Could you check a few things on this model? Use its own coordinates, in mm. Face numbers are marked on the shaded views. Give positions to 0.01 mm unless a question says otherwise; leave off trailing zeros. Loops run counter-clockwise (first coordinate to the right, second up) from the corner with the lowest first, then second, coordinate; pieces in that order, holes last.
1. Imagine slicing it at A-A (z = 0). List the corners of the cut face in (x, y) for me.
2. Imagine slicing it at C-C (x = -47.5). List the corners of the cut face in (y, z) for me, plus the area to 3 significant figures.
3. I need wall thicknesses on line 1 along X through (y, z) = (17.5, 16.7); line 2 along X through (y, z) = (16.6, -61.5); line 3 along Y through (x, z) = (-8, -17.05). Which ranges of each line are inside material? Lowest first, please.
4. Imagine slicing it at B-B (x = -27). List the corners of the cut face in (y, z) for me, plus the area to 3 significant figures.
5. For P1, Ø10, axis at y = 10.5, z = -67.5, coming from the -X side; P2, Ø5, axis at x = -3, y = 16.5, coming from the +Z side; P3, Ø1.4, axis at x = -8, y = 17.5, coming from the +Z side; P4, Ø2, axis at x = 8.5, y = 11.5, coming from the -Z side, each with a flat end and sliding along its axis, tell me the tip position at first contact or that it passes through.
6. Thinking about a two-plate mould opening in Z: for the marked faces 1 and 2, which applies, +Z half, -Z half, draft (parallel to the pull), parting line (faces both ways), or undercut?
7. Imagine slicing it at D-D (x = 58.5). List the corners of the cut face in (y, z) for me.
```python
from build123d import *

# Parameters (mm, degrees)
SKETCH1_R                                           = 37.65
SKETCH1_R_2                                         = 32.65
BOSS_EXTRUDE1_DEPTH                                 = 10
BOSS_EXTRUDE2_START                                 = -4
SKETCH2_R                                           = 32.65
SKETCH2_R_2                                         = 29.65
BOSS_EXTRUDE2_DEPTH                                 = 4
SKETCH3_R                                           = 85
BOSS_EXTRUDE3_DEPTH                                 = 5
SKETCH4_W                                           = 27
SKETCH4_H                                           = 6
BOSS_EXTRUDE4_DEPTH                                 = 6
FILLET1_R                                           = 3
SKETCH6_R                                           = 2.25
CUT_EXTRUDE1_DEPTH                                  = 3
CSK_FOR_M2_COUNTERSUNK_FLAT_HEAD_SCREW1_D           = 2.4
CSK_FOR_M2_COUNTERSUNK_FLAT_HEAD_SCREW1_CSINK_D     = 4.4
CSK_FOR_M2_COUNTERSUNK_FLAT_HEAD_SCREW1_CSINK_ANGLE = 90
FILLET1_OF_MIRROR1_R                                = 3
SKETCH8_R                                           = 2.25
CUT_EXTRUDE2_DEPTH                                  = 5
SKETCH11_W                                          = 6
SKETCH11_H                                          = 16
BOSS_EXTRUDE5_DEPTH                                 = 3
CSK_FOR_M2_COUNTERSUNK_FLAT_HEAD_SCREW2_D           = 2.4
CSK_FOR_M2_COUNTERSUNK_FLAT_HEAD_SCREW2_CSINK_D     = 4.4
CSK_FOR_M2_COUNTERSUNK_FLAT_HEAD_SCREW2_CSINK_ANGLE = 90
LPATTERN1_COUNT                                     = 2
LPATTERN1_PITCH                                     = 16
LPATTERN1_COPY_1_SKETCH_R                           = 2.25
LPATTERN1_COPY_1_DEPTH                              = 5
LPATTERN1_COPY_2_SKETCH_W                           = 6
LPATTERN1_COPY_2_SKETCH_H                           = 16
LPATTERN1_COPY_2_DEPTH                              = 3
LPATTERN1_COPY_3_D                                  = 2.4
LPATTERN1_COPY_3_CSINK_D                            = 4.4
LPATTERN1_COPY_3_CSINK_ANGLE                        = 90
CUT_EXTRUDE3_DEPTH                                  = 122.140414396
CUT_EXTRUDE3_DEPTH_BACK                             = 122.140414396
SKETCH12_R                                          = 12


with BuildPart() as part:
    # Sketch1 → Boss-Extrude1 (new body)
    with BuildSketch(Plane(origin=(0, 0, 0), x_dir=(1, 0, 0), z_dir=(0, 1, 0))):
        with Locations(Location((0, 0, 0), (0, 0, 270))):
            Circle(SKETCH1_R)
        with Locations(Location((0, 0, 0), (0, 0, 270))):
            Circle(SKETCH1_R_2, mode=Mode.SUBTRACT)
    extrude(amount=BOSS_EXTRUDE1_DEPTH)

    # Sketch2 → Boss-Extrude2 (add)
    with BuildSketch(Plane(origin=(0, 10, 0), x_dir=(1, 0, 0), z_dir=(0, 1, 0)).offset(BOSS_EXTRUDE2_START)):
        with Locations(Location((0, 0, 0), (0, 0, 270))):
            Circle(SKETCH2_R)
        with Locations(Location((0, 0, 0), (0, 0, 270))):
            Circle(SKETCH2_R_2, mode=Mode.SUBTRACT)
    extrude(amount=BOSS_EXTRUDE2_DEPTH)

    # Sketch3 → Boss-Extrude3 (add)
    with BuildSketch(Plane(origin=(0, 10, 0), x_dir=(1, 0, 0), z_dir=(0, 1, 0))):
        with Locations(Location((0, 0, 0), (0, 0, 270))):
            Circle(SKETCH3_R)
    extrude(amount=BOSS_EXTRUDE3_DEPTH)

    # Sketch4 → Boss-Extrude4 (add)
    with BuildSketch(Plane(origin=(0, 15, 0), x_dir=(1, 0, 0), z_dir=(0, 1, 0))):
        with Locations((0, 19)):
            Rectangle(SKETCH4_W, SKETCH4_H)
    boss_extrude4 = extrude(amount=BOSS_EXTRUDE4_DEPTH)

    # Fillet1
    fillet1_edges = [part.edges().sort_by_distance(p)[0] for p in [
        (-13.5, 21, -19),
        (13.5, 21, -19),
    ]]
    fillet(fillet1_edges, radius=FILLET1_R)

    # Sketch6 → Cut-Extrude1 (cut)
    with BuildSketch(Plane(origin=(0, 0, -22), x_dir=(-1, 0, 0), z_dir=(0, 0, -1))):
        with Locations((-8, 17.5)):
            Circle(SKETCH6_R)
        with Locations((8, 17.5)):
            Circle(SKETCH6_R)
    cut_extrude1 = extrude(amount=-CUT_EXTRUDE1_DEPTH, mode=Mode.SUBTRACT)

    # CSK for M2 Countersunk Flat Head Screw1 (through all)
    with Locations(Plane(origin=(8, 17.5, -19), x_dir=(-1, 0, 0), z_dir=(0, 0, -1))):
        with Locations((0, 0), (16, 0)):
            csk_for_m2_countersunk_flat_head_screw1 = CounterSinkHole(CSK_FOR_M2_COUNTERSUNK_FLAT_HEAD_SCREW1_D / 2, CSK_FOR_M2_COUNTERSUNK_FLAT_HEAD_SCREW1_CSINK_D / 2, counter_sink_angle=CSK_FOR_M2_COUNTERSUNK_FLAT_HEAD_SCREW1_CSINK_ANGLE)

    # Mirror1: Boss-Extrude4, Cut-Extrude1, CSK for M2 Countersunk Flat Head Screw1 across plane
    add(boss_extrude4.mirror(Plane.XY))
    add(cut_extrude1.mirror(Plane.XY), mode=Mode.SUBTRACT)
    add(csk_for_m2_countersunk_flat_head_screw1.mirror(Plane.XY), mode=Mode.SUBTRACT)

    # Fillet1 of Mirror1
    fillet1_of_mirror1_edges = [part.edges().sort_by_distance(p)[0] for p in [
        (-13.5, 21, 19),
        (13.5, 21, 19),
    ]]
    fillet(fillet1_of_mirror1_edges, radius=FILLET1_OF_MIRROR1_R)

    # Sketch8 → Cut-Extrude2 (cut)
    with BuildSketch(Plane(origin=(0, 10, 0), x_dir=(-1, 0, 0), z_dir=(0, -1, 0))):
        with Locations(Location((13.5, 61.5, 0), (0, 0, 90))):
            Circle(SKETCH8_R)
    cut_extrude2 = extrude(amount=-CUT_EXTRUDE2_DEPTH, mode=Mode.SUBTRACT)

    # Sketch11 → Boss-Extrude5 (add)
    with BuildSketch(Plane(origin=(0, 15, 0), x_dir=(1, 0, 0), z_dir=(0, 1, 0))):
        with Locations((-13.5, 58.5)):
            Rectangle(SKETCH11_W, SKETCH11_H)
    boss_extrude5 = extrude(amount=BOSS_EXTRUDE5_DEPTH)

    # CSK for M2 Countersunk Flat Head Screw2 (through all)
    with Locations(Plane(origin=(-13.5, 15, -61.5), x_dir=(0, 0, -1), z_dir=(0, -1, 0))):
        with Locations((0, 0)):
            csk_for_m2_countersunk_flat_head_screw2 = CounterSinkHole(CSK_FOR_M2_COUNTERSUNK_FLAT_HEAD_SCREW2_D / 2, CSK_FOR_M2_COUNTERSUNK_FLAT_HEAD_SCREW2_CSINK_D / 2, counter_sink_angle=CSK_FOR_M2_COUNTERSUNK_FLAT_HEAD_SCREW2_CSINK_ANGLE)

    # Mirror2: Cut-Extrude2, Boss-Extrude5, CSK for M2 Countersunk Flat Head Screw2 across plane
    add(cut_extrude2.mirror(Plane(origin=(0, 0, 0), x_dir=(0, 0, 1), z_dir=(1, 0, 0))), mode=Mode.SUBTRACT)
    add(boss_extrude5.mirror(Plane(origin=(0, 0, 0), x_dir=(0, 0, 1), z_dir=(1, 0, 0))))
    add(csk_for_m2_countersunk_flat_head_screw2.mirror(Plane(origin=(0, 0, 0), x_dir=(0, 0, 1), z_dir=(1, 0, 0))), mode=Mode.SUBTRACT)

    # LPattern1: Cut-Extrude2, Boss-Extrude5, CSK for M2 Countersunk Flat Head Screw2 ×2
    with Locations(*[(0, 0, i * LPATTERN1_PITCH) for i in range(1, LPATTERN1_COUNT)]):
        add(cut_extrude2, mode=Mode.SUBTRACT)
        add(boss_extrude5)
        add(csk_for_m2_countersunk_flat_head_screw2, mode=Mode.SUBTRACT)

    # LPattern1 copy 1 sketch → LPattern1 copy 1 (cut)
    with BuildSketch(Plane(origin=(0, 10, 16), x_dir=(1, 0, 0), z_dir=(0, -1, 0))):
        with Locations((13.5, -61.5)):
            Circle(LPATTERN1_COPY_1_SKETCH_R)
    extrude(amount=-LPATTERN1_COPY_1_DEPTH, mode=Mode.SUBTRACT)

    # LPattern1 copy 2 sketch → LPattern1 copy 2 (add)
    with BuildSketch(Plane(origin=(0, 15, 16), x_dir=(-1, 0, 0), z_dir=(0, 1, 0))):
        with Locations((-13.5, -58.5)):
            Rectangle(LPATTERN1_COPY_2_SKETCH_W, LPATTERN1_COPY_2_SKETCH_H)
    extrude(amount=LPATTERN1_COPY_2_DEPTH)

    # LPattern1 copy 3 (through all)
    with Locations(Plane(origin=(13.5, 15, -45.5), x_dir=(0, 0, -1), z_dir=(0, -1, 0))):
        with Locations((0, 0)):
            CounterSinkHole(LPATTERN1_COPY_3_D / 2, LPATTERN1_COPY_3_CSINK_D / 2, counter_sink_angle=LPATTERN1_COPY_3_CSINK_ANGLE)

    # Sketch12 → Cut-Extrude3 (cut, two sides: drawn at the far end of the back side and taken through both)
    with BuildSketch(Plane(origin=(0, 15, 0), x_dir=(1, 0, 0), z_dir=(0, 1, 0)).offset(-CUT_EXTRUDE3_DEPTH_BACK)):
        with Locations(Location((0, 68, 0), (0, 0, 270))):
            Circle(SKETCH12_R)
    extrude(amount=CUT_EXTRUDE3_DEPTH + CUT_EXTRUDE3_DEPTH_BACK, mode=Mode.SUBTRACT)


solid = part.part
```
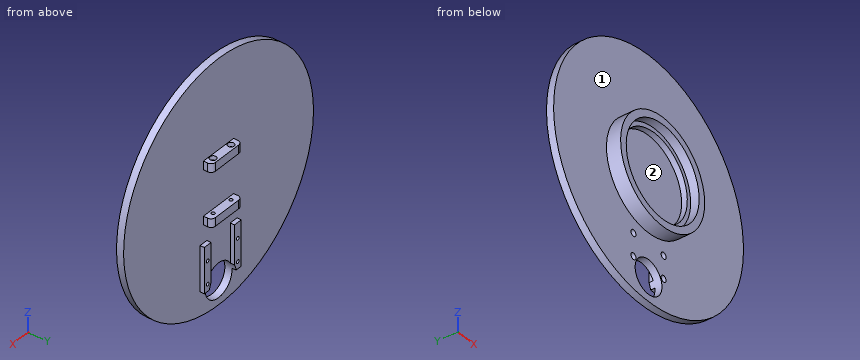
Derived:
1. outline: (-85, 10) - (-37.65, 10) - (-37.65, 0) - (-32.65, 0) - (-32.65, 6) - (-29.65, 6) - (-29.65, 10) - (29.65, 10) - (29.65, 6) - (32.65, 6) - (32.65, 0) - (37.65, 0) - (37.65, 10) - (85, 10) - (85, 15) - (-85, 15) - close
2. outline: (10, -70.49) - (15, -70.49) - (15, 70.49) - (10, 70.49) - close
2. area: 705 mm2
3. line 1: x = -13.5 to -9.2, -6.8 to 6.8, 9.2 to 13.5
3. line 2: x = -16.5 to -14.7, -12.3 to -10.5, 10.5 to 12.3, 14.7 to 16.5
3. line 3: y = 10 to 16.3, 18.7 to 21
4. outline: (0, -26.24) - (10, -26.24) - (10, -80.6) - (15, -80.6) - (15, 80.6) - (10, 80.6) - (10, 26.24) - (0, 26.24) - (0, 18.36) - (6, 18.36) - (6, 12.25) - (10, 12.25) - (10, -12.25) - (6, -12.25) - (6, -18.36) - (0, -18.36) - close
4. area: 1,010 mm2
5. P1: stops at x = -57.61
5. P2: stops at z = 84.99
5. P3: passes through
5. P4: stops at z = -84.67
6. face 1: draft
6. face 2: undercut
7. outline: (10, -61.67) - (15, -61.67) - (15, 61.67) - (10, 61.67) - close
